For this review, take the finished solid that the model builds, in its own axes (mm). A direction names the side the tool comes from. Round coordinates to 2 decimals unless told otherwise and drop trailing zeros.
1. Draft analysis for pull direction Z (two halves, no side actions). For faces 1 (the flat face through (-45, 10, 0)), 2 (the flat face through (-10, 10, 25)), 3 (the flat face through (-23, 12.7, -20)), 4 (the flat face through (-10, 10, -25)), state which applies: released by +Z, released by -Z, zero draft, split by the parting line, or undercut.
2. Tool access review of faces 5 (the flat face through (19.11, 13.87, -20.14)), 6 (the flat face through (-10, 0, 0)): name each direction out of +Z, -Z, +X, -X, +Y, -Y from which nothing blocks a thin tool from reaching the whole face with its end or side.
3. To check wall thickness, follow line 1 along Z through (x, y) = (21.5, 16.6); line 2 along X through (y, z) = (17.05, 21.5). State the ranges of each line that lie inside material, in increasing order.
4. Clearance check with a flat-ended pin moving along its axis: pin 1 Ø3.5 at (x, z) = (21.5, 21.5) entering from -Y. State where the tip first meets the part, or that it passes through.
from build123d import *

# Parameters (mm, degrees)
SKETCH1_W           = 50
SKETCH1_H           = 50
SKETCH1_R           = 1.6
BOSS_EXTRUDE1_DEPTH = 20
CUT_EXTRUDE1_START  = -5
CUT_EXTRUDE1_DEPTH  = 2.3
SKETCH3_W           = 50
SKETCH3_H           = 20
BOSS_EXTRUDE2_DEPTH = 20


with BuildPart() as part:
    # Sketch1 → Boss-Extrude1 (new body)
    with BuildSketch(Plane(origin=(0, 0, 0), x_dir=(1, 0, 0), z_dir=(0, 1, 0))):
        Rectangle(SKETCH1_W, SKETCH1_H)
        with Locations(Location((21.5, 21.5, 0), (0, 0, 270))):
            Circle(SKETCH1_R, mode=Mode.SUBTRACT)
        with Locations(Location((21.5, -21.5, 0), (0, 0, 270))):
            Circle(SKETCH1_R, mode=Mode.SUBTRACT)
        with Locations(Location((-21.5, -21.5, 0), (0, 0, 270))):
            Circle(SKETCH1_R, mode=Mode.SUBTRACT)
        with Locations(Location((-21.5, 21.5, 0), (0, 0, 270))):
            Circle(SKETCH1_R, mode=Mode.SUBTRACT)
    extrude(amount=BOSS_EXTRUDE1_DEPTH)

    # Sketch2 → Cut-Extrude1 (cut)
    with BuildSketch(Plane(origin=(0, 20, 0), x_dir=(1, 0, 0), z_dir=(0, 1, 0)).offset(CUT_EXTRUDE1_START)):
        Polygon((24.675426481, 21.5), (23.08771324, 24.25), (19.91228676, 24.25), (18.324573519, 21.5), (19.91228676, 18.75), (23.08771324, 18.75), align=None)
        Polygon((-21.5, 24.675426481), (-24.25, 23.08771324), (-24.25, 19.91228676), (-21.5, 18.324573519), (-18.75, 19.91228676), (-18.75, 23.08771324), align=None)
        Polygon((21.5, -24.675426481), (24.25, -23.08771324), (24.25, -19.91228676), (21.5, -18.324573519), (18.75, -19.91228676), (18.75, -23.08771324), align=None)
        Polygon((-24.675426481, -21.5), (-23.08771324, -24.25), (-19.91228676, -24.25), (-18.324573519, -21.5), (-19.91228676, -18.75), (-23.08771324, -18.75), align=None)
    extrude(amount=-CUT_EXTRUDE1_DEPTH, mode=Mode.SUBTRACT)

    # Sketch3 → Boss-Extrude2 (add)
    with BuildSketch(Plane.ZY.offset(25)):
        with Locations((0, 10)):
            Rectangle(SKETCH3_W, SKETCH3_H)
    extrude(amount=BOSS_EXTRUDE2_DEPTH)


solid = part.part
Resolved:
1. face 1: zero draft
1. face 2: released by +Z
1. face 3: undercut
1. face 4: released by -Z
2. face 5: none
2. face 6: +Z, -Z, +X, -X, -Y
3. line 1: z = -25 to -23.1, -19.9 to 19.9, 23.1 to 25
3. line 2: x = -45 to -23.1, -19.9 to 19.9, 23.1 to 25
4. pin 1: stops at y = 0
